```python
from build123d import *

# Parameters (mm, degrees)
F1_DEPTH = 9.525
F2_R     = 1.0795
F3_DEPTH = 4.7498
F4_R     = 1.016
F5_DEPTH = 4.7498


with BuildPart() as f1:
    # F0 (on Top) → F1 (new body)
    with BuildSketch(Plane.XY):
        Polygon((1.833087, -3.175), (3.666174, 0), (1.833087, 3.175), (-1.833087, 3.175), (-3.666174, 0), (-1.833087, -3.175), align=None)
    extrude(amount=F1_DEPTH)

    # F2 (on face) → F3 (join)
    with BuildSketch(Plane(origin=(0, 0, 0), x_dir=(1, 0, 0), z_dir=(0, 0, -1))):
        Circle(F2_R)
    extrude(amount=F3_DEPTH)

    # F4 (on face) → F5 (cut)
    with BuildSketch(Plane.XY.offset(9.525)):
        Circle(F4_R)
    extrude(amount=-F5_DEPTH, mode=Mode.SUBTRACT)


solid = f1.part
```
CAD build for the part. Positions are in the model's coordinates, mm. A direction names the side the tool comes from. Round coordinates to 2 decimals unless told otherwise and drop trailing zeros. Order: outer loops, then holes, each group sorted by start corner. A loop starts at its lowest first (then second) coordinate and runs counter-clockwise, first axis right, second up. Notation, with made-up numbers: (1, 53.5) - (38, 53.5) arc R10 ccw to (38, 68.5) - close; hole circle Ø7 at (64, 27). An arc over 180 degrees is marked (long way). Answer as CSV lines item,"result". Start each with the question number.
1. Saw through at A-A, the plane z = 7.5. Write the cut outline in (x, y) (3 decimals), and give its area (3 significant figures).
2. Saw through at D-D, the plane y = 0.75. Write the cut outline in (x, z) (3 decimals).
3. Saw through at C-C, the plane z = 4.5. Write the cut outline in (x, y) (3 decimals), and give its area (3 significant figures).
4. Tool access for faces 4 (the face through (0, 0, 4.775)), 5 (the face through (-1, -1, 0)), 6 (the face through (2.737, -1.61, 4.696)): list every direction of +Z, -Z, +X, -X, +Y, -Y with a clear straight run to the whole face (end or side of a thin tool).
5. Pin check, flat tips, straight feed: pin 1 (1 mm diameter, centred on y = 1.5, z = 5, fed in from +X); pin 2 (1.6 mm diameter, centred on x = 0, y = 0, fed in from +Z); pin 3 (1.9 mm diameter, centred on x = 2, y = 0.5, fed in from -Z). Stop position of each tip, or through.
6. Saw through at B-B, the plane x = 0. Write the cut outline in (y, z) (1 decimal), and give its area (3 significant figures).
7. Drill centre lines: L1, parallel to Y at x = 0, z = 7.4 (3 decimals); L2, parallel to Z at x = -0.75, y = -3 (3 decimals); L3, parallel to X at y = 0.5, z = -3.5. Where is each one in solid material? Low to high. Write a range as [from, to].
8. Pull direction Y, two halves, no side cores. Call faces 1 (the face through (0, 3.175, 5)), 2 (the face through (-0.22, -0.99, 7.18)), 3 (the face through (0, -3.175, 5)): +Y half, -Y half, draft (parallel to the pull), parting line (faces both ways), or undercut.
Model answer:
1,outline,"(-3.666, 0) - (-1.833, -3.175) - (1.833, -3.175) - (3.666, 0) - (1.833, 3.175) - (-1.833, 3.175) - close; hole circle Ø2.032 at (0, 0)"
1,area,"31.7 mm²"
2,outline,"(-3.233, 0) - (-0.776, 0) - (-0.776, -4.75) - (0.776, -4.75) - (0.776, 0) - (3.233, 0) - (3.233, 9.525) - (0.685, 9.525) - (0.685, 4.775) - (-0.685, 4.775) - (-0.685, 9.525) - (-3.233, 9.525) - close"
3,outline,"(-3.666, 0) - (-1.833, -3.175) - (1.833, -3.175) - (3.666, 0) - (1.833, 3.175) - (-1.833, 3.175) - close"
3,area,"34.9 mm²"
4,face 4,"+Z"
4,face 5,"-Z"
4,face 6,"+Z, -Z, +X, -Y"
5,pin 1,"stops at x = 3.09"
5,pin 2,"stops at z = 4.78"
5,pin 3,"stops at z = 0"
6,outline,"(-3.2, 0) - (-1.1, 0) - (-1.1, -4.7) - (1.1, -4.7) - (1.1, 0) - (3.2, 0) - (3.2, 9.5) - (1, 9.5) - (1, 4.8) - (-1, 4.8) - (-1, 9.5) - (-3.2, 9.5) - close"
6,area,"61.1 mm²"
7,L1,"y = [-3.175, -1.016], [1.016, 3.175]"
7,L2,"z = [0, 9.525]"
7,L3,"x = [-0.96, 0.96]"
8,face 1,"+Y half"
8,face 2,"undercut"
8,face 3,"-Y half"
